```python
from build123d import *

# Parameters (mm, degrees)
F1_DEPTH = 5
F3_DEPTH = 25
F4_DEPTH = 3.2
F5_SIZE  = 0.2
F6_SIZE2 = 0.535898
F6_SIZE  = 2


with BuildPart() as f1:
    # F0 (on Top) → F1 (new body)
    with BuildSketch(Plane.XY):
        with BuildLine():
            Line((-34.477164, 42.681355), (-34.477164, 68.681355))
            ThreePointArc((-34.477164, 68.681355), (-35.004372, 69.954148), (-36.277164, 70.481355))
            Line((-36.277164, 70.481355), (-44.277164, 70.481355))
            ThreePointArc((-44.277164, 70.481355), (-45.549957, 69.954148), (-46.077164, 68.681355))
            Line((-46.077164, 68.681355), (-46.077164, 42.681355))
            ThreePointArc((-46.077164, 42.681355), (-45.549957, 41.408563), (-44.277164, 40.881355))
            Line((-44.277164, 40.881355), (-36.277164, 40.881355))
            ThreePointArc((-36.277164, 40.881355), (-35.004372, 41.408563), (-34.477164, 42.681355))
        make_face()
    extrude(amount=F1_DEPTH)

    # F2 (on face) → F3 (cut)
    with BuildSketch(Plane.XY.offset(5)):
        with BuildLine():
            ThreePointArc((-38.777164, 65.481355), (-39.216504, 66.542015), (-40.277164, 66.981355))
            ThreePointArc((-40.277164, 66.981355), (-41.337825, 64.420695), (-38.777164, 65.481355))
        make_face()
        with BuildLine():
            ThreePointArc((-38.777164, 45.881355), (-41.337825, 46.942015), (-40.277164, 44.381355))
            ThreePointArc((-40.277164, 44.381355), (-39.216504, 44.820695), (-38.777164, 45.881355))
        make_face()
    extrude(amount=-F3_DEPTH, mode=Mode.SUBTRACT)

    # F2 (on face) → F4 (cut)
    with BuildSketch(Plane.XY.offset(5)):
        with BuildLine():
            ThreePointArc((-37.427164, 65.481355), (-38.26191, 67.49661), (-40.277164, 68.331355))
            ThreePointArc((-40.277164, 68.331355), (-42.292419, 63.466101), (-37.427164, 65.481355))
        make_face()
        with BuildLine():
            ThreePointArc((-38.777164, 65.481355), (-41.337825, 64.420695), (-40.277164, 66.981355))
            ThreePointArc((-40.277164, 66.981355), (-39.216504, 66.542015), (-38.777164, 65.481355))
        make_face(mode=Mode.SUBTRACT)
        with BuildLine():
            ThreePointArc((-37.427164, 45.881355), (-42.292419, 47.89661), (-40.277164, 43.031355))
            ThreePointArc((-40.277164, 43.031355), (-38.26191, 43.866101), (-37.427164, 45.881355))
        make_face()
        with BuildLine():
            ThreePointArc((-38.777164, 45.881355), (-39.216504, 44.820695), (-40.277164, 44.381355))
            ThreePointArc((-40.277164, 44.381355), (-41.337825, 46.942015), (-38.777164, 45.881355))
        make_face(mode=Mode.SUBTRACT)
    extrude(amount=-F4_DEPTH, mode=Mode.SUBTRACT)

    # F5
    f5_edges = [f1.edges().sort_by_distance(p)[0] for p in [
        (-41.777164, 65.481355, 1.8),
        (-40.277164, 47.381355, 1.8),
        (-34.477164, 55.681355, 0),
        (-35.004372, 41.408563, 0),
        (-35.004372, 69.954148, 0),
        (-40.277164, 40.881355, 0),
        (-40.277164, 70.481355, 0),
        (-45.549957, 41.408563, 0),
        (-45.549957, 69.954148, 0),
        (-46.077164, 55.681355, 0),
        (-40.277164, 47.381355, 0),
        (-41.777164, 65.481355, 0),
        (-43.127164, 65.481355, 5),
        (-40.277164, 48.731355, 5),
    ]]
    chamfer(f5_edges, length=F5_SIZE)

    # F6
    f6_edges = [f1.edges().sort_by_distance(p)[0] for p in [
        (-34.477164, 55.681355, 5),
    ]]
    chamfer(f6_edges, length=F6_SIZE, length2=F6_SIZE2)


solid = f1.part
```
Read the model definition and answer for the solid it produces. Units are mm, in the model's axes. A direction names the side the tool comes from. Coordinates: 2 decimals unless noted, no trailing zeros. Loops run counter-clockwise (first coordinate to the right, second up) from the corner with the lowest first, then second, coordinate; pieces in that order, holes last. Notation, with made-up numbers: (47.25, 89.25) -> (68.25, 89.25) arc R22 ccw to (68.25, 117.25) -> close; hole circle Ø2 at (13, 65). An arc over 180 degrees is marked (long way). Return JSON: item names as keys, results as strings.
Item 1: Find section C-C (z = 1). Determine the outline of the cut face in (x, y).
Answers:
{"outline": "(-46.08, 42.68) arc R1.8 ccw to (-44.28, 40.88) -> (-36.28, 40.88) arc R1.8 ccw to (-34.48, 42.68) -> (-34.48, 68.68) arc R1.8 ccw to (-36.28, 70.48) -> (-44.28, 70.48) arc R1.8 ccw to (-46.08, 68.68) -> close; hole circle Ø3 at (-40.28, 45.88); hole circle Ø3 at (-40.28, 65.48)"}
Item 2: Find section B-B (y = 56.75). Determine the outline of the cut face in (x, z), plus the area to 3 significant figures.
Answers:
{"outline": "(-46.08, 0.2) -> (-45.88, 0) -> (-34.68, 0) -> (-34.48, 0.2) -> (-34.48, 3) -> (-35.01, 5) -> (-45.54, 5) -> (-46.08, 3) -> close", "area": "56.9 mm2"}
Item 3: Flat-ended cylindrical pins translate along their axes: P1, Ø2.5, axis at x = -40.28, y = 45.88, coming from the +Z side; P2, Ø3, axis at x = -39.5, y = 66.5, coming from the +Z side. Find the tip coordinate at first contact, or state that the pin passes through.
Answers:
{"P1": "passes through", "P2": "stops at z = 1.8"}
Item 4: Find section A-A (z = 2.3). Determine the outline of the cut face in (x, y).
Answers:
{"outline": "(-46.08, 42.68) arc R1.8 ccw to (-44.28, 40.88) -> (-36.28, 40.88) arc R1.8 ccw to (-34.48, 42.68) -> (-34.48, 68.68) arc R1.8 ccw to (-36.28, 70.48) -> (-44.28, 70.48) arc R1.8 ccw to (-46.08, 68.68) -> close; hole circle Ø5.7 at (-40.28, 45.88); hole circle Ø5.7 at (-40.28, 65.48)"}
Item 5: Find the intervals of material crossed by probe 1 along X at (y, z) = (65.5, 1.95); probe 2 along Y at (x, z) = (-41.25, 2.05); probe 3 along Y at (x, z) = (-41.5, 3.3), in increasing order.
Answers:
{"probe 1": "x = -46.08 to -43.13, -37.43 to -34.48", "probe 2": "y = 40.88 to 43.2, 48.56 to 62.8, 68.16 to 70.48", "probe 3": "y = 40.96 to 43.31, 48.46 to 62.91, 68.06 to 70.4"}
Item 6: For a pull along Y with two mould halves and no side action, classify faces 3 (the flat face through (-40, 44, 1.8)), 4 (the flat face through (-40, 56, 0)), 5 (the flat face through (-40.33, 41.15, 4.01)) as +Y half, -Y half, draft (parallel to the pull), parting line (faces both ways), or undercut.
Answers:
{"face 3": "undercut", "face 4": "draft", "face 5": "-Y half"}
Item 7: Find section D-D (x = -39.5). Count the separate pieces of the cut face and the enclosed holes in it, plus the area to 3 significant figures.
Answers:
{"separate pieces": "3", "enclosed holes": "0", "area": "102 mm2"}
Item 8: For faces 1 (the flat face through (-39, 64, 1.8)), 2 (the cylindrical face through (-34.99, 69.94, 1.58)), determine the directions among +Z, -Z, +X, -X, +Y, -Y from which every point of the face is accessible in a straight line to the end or side of a thin tool.
Answers:
{"face 1": "+Z", "face 2": "+Z, -Z, +X, +Y"}
